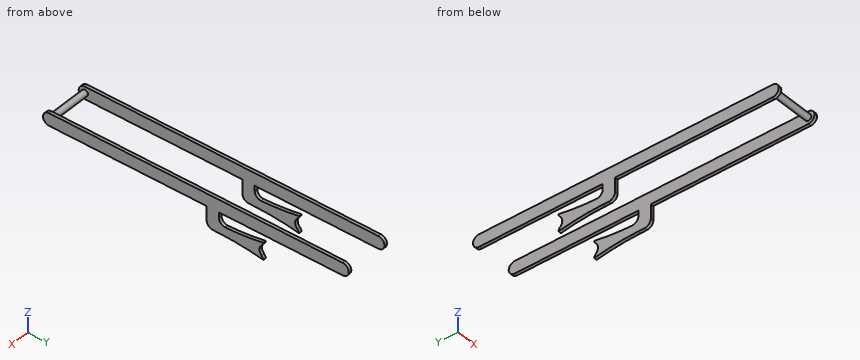
```python
from build123d import *

# Parameters (mm, degrees)
SKETCH_1_W        = 10
SKETCH_1_H        = 40
EXTRUDE_1_DEPTH   = 950
EXTRUDE_1_2_DEPTH = 950
SKETCH_2_R        = 10
EXTRUDE_2_DEPTH   = 150
SKETCH_3_R        = 20
EXTRUDE_3_DEPTH   = 10
EXTRUDE_START     = -10
SKETCH_4_R        = 20
EXTRUDE_4_DEPTH   = 10
EXTRUDE_5_DEPTH   = 10
EXTRUDE_6_DEPTH   = 10
FILLET_1_R        = 20


with BuildPart() as part:
    # Sketch 1 → Extrude 1 (new body)
    with BuildSketch(Plane(origin=(0, 0, 0), x_dir=(1, 0, 0), z_dir=(0, 1, 0))):
        with Locations((-70, 0)):
            Rectangle(SKETCH_1_W, SKETCH_1_H)
    extrude(amount=EXTRUDE_1_DEPTH)



with BuildPart() as body_2:
    # Sketch 1 → Extrude 1 2 (new body)
    with BuildSketch(Plane(origin=(0, 0, 0), x_dir=(1, 0, 0), z_dir=(0, 1, 0))):
        with Locations((70, 0)):
            Rectangle(SKETCH_1_W, SKETCH_1_H)
    extrude(amount=EXTRUDE_1_2_DEPTH)


with BuildPart() as part_1:
    add(part.part)

    add(body_2.part)  # Extrude 2 merges body 2
    # Sketch 2 → Extrude 2 (add)
    with BuildSketch(Plane(origin=(75, 0, 0), x_dir=(0, 0, -1), z_dir=(1, 0, 0))):
        Circle(SKETCH_2_R)
    extrude(amount=-EXTRUDE_2_DEPTH)

    # Sketch 3 → Extrude 3 (add)
    with BuildSketch(Plane(origin=(75, 0, 0), x_dir=(0, 0, -1), z_dir=(1, 0, 0))):
        with Locations((0, 950)):
            Circle(SKETCH_3_R)
        Circle(SKETCH_3_R)
    extrude(amount=-EXTRUDE_3_DEPTH)

    # Sketch 4 → Extrude 4 (add)
    with BuildSketch(Plane.ZY.offset(75).offset(EXTRUDE_START)):
        with Locations((0, 950)):
            Circle(SKETCH_4_R)
        Circle(SKETCH_4_R)
    extrude(amount=EXTRUDE_4_DEPTH)

    # Sketch 5 → Extrude 5 (add)
    with BuildSketch(Plane.ZY.offset(75)):
        with BuildLine():
            Line((-1.961717338, 550), (-58.000349557, 550))
            ThreePointArc((-58.000349557, 550), (-54.659475196, 622.066890367), (-44.665509494, 693.515604688))
            Line((-44.665509494, 693.515604688), (-52.51833449, 691.655753978))
            ThreePointArc((-52.51833449, 691.655753978), (-71.961717338, 680.941793153), (-91.405100186, 691.655753978))
            Line((-91.405100186, 691.655753978), (-99.257925182, 693.515604688))
            ThreePointArc((-99.257925182, 693.515604688), (-89.26395948, 622.066890367), (-85.923085118, 550))
            Line((-85.923085118, 550), (-85.923085118, 510))
            Line((-85.923085118, 510), (-1.961717338, 510))
            Line((-1.961717338, 510), (-1.961717338, 550))
        make_face()
    extrude(amount=-EXTRUDE_5_DEPTH)

    # Sketch 6 → Extrude 6 (add)
    with BuildSketch(Plane.ZY.offset(-65)):
        with BuildLine():
            Line((-1.961717338, 550), (-58.000349557, 550))
            ThreePointArc((-58.000349557, 550), (-54.659475196, 622.066890367), (-44.665509494, 693.515604688))
            Line((-44.665509494, 693.515604688), (-52.51833449, 691.655753978))
            ThreePointArc((-52.51833449, 691.655753978), (-71.961717338, 680.941793153), (-91.405100186, 691.655753978))
            Line((-91.405100186, 691.655753978), (-99.257925182, 693.515604688))
            ThreePointArc((-99.257925182, 693.515604688), (-89.26395948, 622.066890367), (-85.923085118, 550))
            Line((-85.923085118, 550), (-85.923085118, 510))
            Line((-85.923085118, 510), (-1.961717338, 510))
            Line((-1.961717338, 510), (-1.961717338, 550))
        make_face()
    extrude(amount=-EXTRUDE_6_DEPTH)

    # Fillet 1
    fillet_1_edges = [part_1.edges().sort_by_distance(p)[0] for p in [
        (70, 550, -58.000349557),
        (70, 510, -85.923085118),
        (70, 691.655753978, -91.405100186),
        (70, 691.655753978, -52.51833449),
        (-70, 550, -58.000349557),
        (-70, 510, -85.923085118),
        (-70, 691.655753978, -91.405100186),
        (-70, 691.655753978, -52.51833449),
    ]]
    fillet(fillet_1_edges, radius=FILLET_1_R)


solid = part_1.part
```
The listing builds one solid part. Answer for the finished solid, in the listing's coordinates (mm). Round coordinates to 2 decimals unless told otherwise and drop trailing zeros. Loops run counter-clockwise (first coordinate to the right, second up) from the corner with the lowest first, then second, coordinate; pieces in that order, holes last.
Q1. Find the intervals of material crossed by line 1 (X direction, y = 644.5, z = -7); line 2 (Y direction, x = 63, z = -5); line 3 (Y direction, x = 68.5, z = -71), in increasing order.
Q2. Section C-C, the plane z = -77.5 is taken. Determine the outline of the cut face in (x, y).
Q3. Given pin 1 Ø11 at (x, z) = (70.5, -46) entering from -Y; pin 2 Ø8 at (x, z) = (68.5, -32) entering from +Y; pin 3 Ø3 at (x, y) = (67.5, 203.5) entering from -Z, each flat-ended and moving along its own axis, determine where each tip first touches the part or whether it passes through.
Q4. Section B-B, the plane z = 0 is taken. Determine the outline of the cut face in (x, y).
Q5. Section A-A, the plane y = 125 is taken. Determine the outline of the cut face in (x, z).
Q6. Section D-D, the plane x = -48 is taken. Determine the outline of the cut face in (y, z).
Completed:
1. line 1: x = -75 to -65, 65 to 75
1. line 2: y = -8.66 to 8.66
1. line 3: y = 510.66 to 680.96
2. outline: (-75, 513.69) - (-65, 513.69) - (-65, 681.62) - (-75, 681.62) - close; (65, 513.69) - (75, 513.69) - (75, 681.62) - (65, 681.62) - close
3. pin 1: stops at y = 510
3. pin 2: stops at y = 550
3. pin 3: stops at z = -20
4. outline: (-75, -20) - (-65, -20) - (-65, -10) - (65, -10) - (65, -20) - (75, -20) - (75, 970) - (65, 970) - (65, 10) - (-65, 10) - (-65, 970) - (-75, 970) - close
5. outline: (-75, -20) - (-65, -20) - (-65, 20) - (-75, 20) - close; (65, -20) - (75, -20) - (75, 20) - (65, 20) - close
6. outline: circle Ø20 at (0, 0)
